from build123d import *

# Parameters (mm, degrees)
F0_W     = 30
F0_H     = 9.55
F0_H_2   = 2
F0_H_3   = 11.15
F0_W_2   = 1.5
F0_W_3   = 20.75
F1_DEPTH = 2
F2_DEPTH = 8.5
F3_D     = 3.2


with BuildPart() as f1:
    # F0 (on Top) → F1 (new body)
    with BuildSketch(Plane.XY):
        with Locations((0, 17.925)):
            Rectangle(F0_W, F0_H)
        with Locations((0, 12.15)):
            Rectangle(F0_W, F0_H_2)
        with Locations((0, 5.575)):
            Rectangle(F0_W, F0_H_3)
        with Locations((0, -1)):
            Rectangle(F0_W, F0_H_2)
        with Locations((-36.5, 5.575)):
            Rectangle(F0_W_2, F0_H_3)
        with Locations((-25.375, 5.575)):
            Rectangle(F0_W_3, F0_H_3)
        with Locations((25.375, 5.575)):
            Rectangle(F0_W_3, F0_H_3)
        with Locations((36.5, 5.575)):
            Rectangle(F0_W_2, F0_H_3)
    extrude(amount=F1_DEPTH)

    # F0 (on Top) → F2 (join)
    with BuildSketch(Plane.XY):
        with Locations((0, 12.15)):
            Rectangle(F0_W, F0_H_2)
        with Locations((0, -1)):
            Rectangle(F0_W, F0_H_2)
        with Locations((-36.5, 5.575)):
            Rectangle(F0_W_2, F0_H_3)
        with Locations((36.5, 5.575)):
            Rectangle(F0_W_2, F0_H_3)
    extrude(amount=F2_DEPTH)

    # F3 (through all)
    with Locations(Plane(origin=(0, 0, 0), x_dir=(1, 0, 0), z_dir=(0, 0, -1))):
        with Locations((0, -17.7)):
            Hole(F3_D / 2)


solid = f1.part
Check sheet for the modelled part. Datum: model origin and axes. Units: mm. A direction names the side the tool comes from. Round coordinates to 2 decimals unless told otherwise and drop trailing zeros. Loops run counter-clockwise (first coordinate to the right, second up) from the corner with the lowest first, then second, coordinate; pieces in that order, holes last.
1. Sectioned sample at C-C on x = 0. Record the boundary of the cut face in (y, z), and give its area (3 significant figures).
2. Sectioned sample at D-D on y = 3.5. Record the boundary of the cut face in (x, z), and give its area (4 significant figures).
3. Mould release check, pull along X, two halves, no side actions. Record for faces 1 (the flat face through (0, 11.15, 5)), 2 (the flat face through (0, 12, 8.5)), 3 (the flat face through (-37.25, 5, 4)): released by +X, released by -X, zero draft, split by the parting line, or undercut.
4. Set-up check for faces 4 (the flat face through (15, 14, 1)), 5 (the flat face through (35.75, 5, 5)), 6 (the flat face through (0, 20, 2)), 7 (the flat face through (-1, 6, 2)): record each of +Z, -Z, +X, -X, +Y, -Y from which the full face is reachable in a straight line by a thin tool's end or side.
5. Sectioned sample at A-A on y = 17.7. Record the boundary of the cut face in (x, z), and give its area (3 significant figures).
6. Sectioned sample at B-B on z = 7.5. Record the boundary of the cut face in (x, y).
7. Gauge pin test, flat ends, axial feed: pin 1 Ø4 at (x, z) = (-26, 2.5) entering from -Y; pin 2 Ø7.5 at (x, y) = (1.5, 15.5) entering from +Z; pin 3 Ø4 at (y, z) = (19.5, 3.5) entering from -X; pin 4 Ø2 at (x, z) = (5.5, 5) entering from +Y. Record the tip position at first contact, or that the pin passes through.
8. Scan lines: probe 1 along Y at (x, z) = (0, 0.7); probe 2 along Y at (x, z) = (9.5, 2.75); probe 3 along X at (y, z) = (17.7, 1.3). Record each from-to range of solid material in increasing order.
Recorded:
1. outline: (-2, 0) - (16.1, 0) - (16.1, 2) - (13.15, 2) - (13.15, 8.5) - (11.15, 8.5) - (11.15, 2) - (0, 2) - (0, 8.5) - (-2, 8.5) - close; (19.3, 0) - (22.7, 0) - (22.7, 2) - (19.3, 2) - close
1. area: 69.0 mm2
2. outline: (-37.25, 0) - (37.25, 0) - (37.25, 8.5) - (35.75, 8.5) - (35.75, 2) - (-35.75, 2) - (-35.75, 8.5) - (-37.25, 8.5) - close
2. area: 168.5 mm2
3. face 1: undercut
3. face 2: zero draft
3. face 3: released by -X
4. face 4: +Z, -Z, +X, +Y
4. face 5: +Z, +Y, -Y
4. face 6: +Z, +X, -X, +Y
4. face 7: +Z
5. outline: (-15, 0) - (-1.6, 0) - (-1.6, 2) - (-15, 2) - close; (1.6, 0) - (15, 0) - (15, 2) - (1.6, 2) - close
5. area: 53.6 mm2
6. outline: (-37.25, 0) - (-35.75, 0) - (-35.75, 11.15) - (-37.25, 11.15) - close; (-15, -2) - (15, -2) - (15, 0) - (-15, 0) - close; (-15, 11.15) - (15, 11.15) - (15, 13.15) - (-15, 13.15) - close; (35.75, 0) - (37.25, 0) - (37.25, 11.15) - (35.75, 11.15) - close
7. pin 1: stops at y = 0
7. pin 2: stops at z = 8.5
7. pin 3: stops at x = -15
7. pin 4: stops at y = 13.15
8. probe 1: y = -2 to 16.1, 19.3 to 22.7
8. probe 2: y = -2 to 0, 11.15 to 13.15
8. probe 3: x = -15 to -1.6, 1.6 to 15
